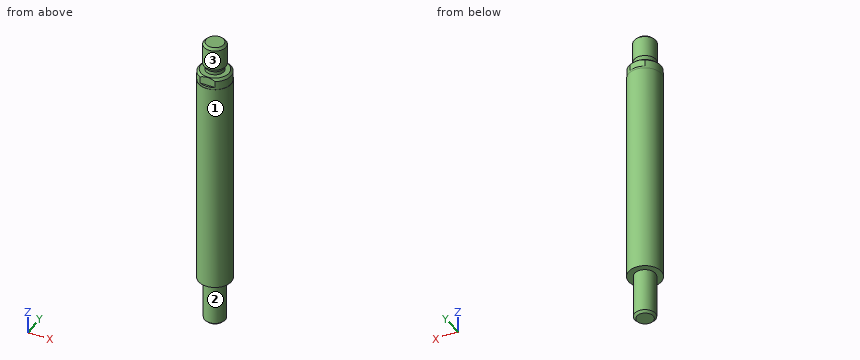
from build123d import *

# Parameters (mm, degrees)
ESQUISSE1_R                   = 15
TIGE_DEPTH                    = 277
ESQUISSE2_OUTSIDE_W           = 88.046
ESQUISSE2_OUTSIDE_H           = 88.046
ESQUISSE2_OUTSIDE_R           = 14.75
CENTRAGE_DE_CHAPE_DEPTH       = 37
ESQUISSE3_OUTSIDE_W           = 88.046
ESQUISSE3_OUTSIDE_H           = 88.046
ESQUISSE3_OUTSIDE_R           = 10
DIAM_TRE_DE_FILETAGE_DEPTH    = 27
ESQUISSE4_OUTSIDE_W           = 88.046
ESQUISSE4_OUTSIDE_H           = 88.046
ESQUISSE4_OUTSIDE_R           = 8.25
GORGE_DE_D_GAGEMENT_DEPTH     = 3
ESQUISSE5_OUTSIDE_W           = 91.51
ESQUISSE5_OUTSIDE_H           = 91.51
ESQUISSE5_OUTSIDE_R           = 8.25
CHANFREIN_DE_D_GAGEMENT_DEPTH = 3
CHANFREIN_DE_D_GAGEMENT_DRAFT = -30
CHANFREIN4_SIZE               = 2
M_PLAT_1_REACH                = 280.815
ESQUISSE6_W                   = 29.5
ESQUISSE6_H                   = 8
ESQUISSE7_OUTSIDE_W           = 88.046
ESQUISSE7_OUTSIDE_H           = 88.046
ESQUISSE7_OUTSIDE_R           = 9.5
CENTRAGE_DE_PISTON_DEPTH      = 42
CHANFREIN_DE_FILETAGE_SIZE    = 2


with BuildPart() as part:
    # Esquisse1 → tige (new body)
    with BuildSketch(Plane.XY):
        with Locations(Location((0, 0, 0), (0, 0, 180))):
            Circle(ESQUISSE1_R)
    extrude(amount=TIGE_DEPTH)

    # Esquisse2 outside → centrage de chape (cut)
    with BuildSketch(Plane.XY.offset(277)):
        Rectangle(ESQUISSE2_OUTSIDE_W, ESQUISSE2_OUTSIDE_H)
        Circle(ESQUISSE2_OUTSIDE_R, mode=Mode.SUBTRACT)
    extrude(amount=-CENTRAGE_DE_CHAPE_DEPTH, mode=Mode.SUBTRACT)

    # Esquisse3 outside → diamètre de filetage (cut)
    with BuildSketch(Plane.XY.offset(277)):
        Rectangle(ESQUISSE3_OUTSIDE_W, ESQUISSE3_OUTSIDE_H)
        Circle(ESQUISSE3_OUTSIDE_R, mode=Mode.SUBTRACT)
    extrude(amount=-DIAM_TRE_DE_FILETAGE_DEPTH, mode=Mode.SUBTRACT)

    # Esquisse4 outside → gorge de d_gagement (cut)
    with BuildSketch(Plane.XY.offset(250)):
        Rectangle(ESQUISSE4_OUTSIDE_W, ESQUISSE4_OUTSIDE_H)
        with Locations(Location((0, 0, 0), (0, 0, 180))):
            Circle(ESQUISSE4_OUTSIDE_R, mode=Mode.SUBTRACT)
    extrude(amount=GORGE_DE_D_GAGEMENT_DEPTH, mode=Mode.SUBTRACT)


with BuildPart() as chanfrein_de_d_gagement_tool:
    # Esquisse5 outside → chanfrein de dégagement (with draft: the straight prism first)
    with BuildSketch(Plane(origin=(0, 0, 253), x_dir=(-1, 0, 0), z_dir=(0, 0, -1))):
        Rectangle(ESQUISSE5_OUTSIDE_W, ESQUISSE5_OUTSIDE_H)
        Circle(ESQUISSE5_OUTSIDE_R, mode=Mode.SUBTRACT)
    extrude(amount=-CHANFREIN_DE_D_GAGEMENT_DEPTH)
    # chanfrein de dégagement: the draft: its side faces are tilted about the plane it starts from
    chanfrein_de_d_gagement_sides = [chanfrein_de_d_gagement_tool.faces().sort_by_distance(p)[0] for p in [
        (0, -45.755, 254.5),
        (-45.755, 0, 254.5),
        (0, 45.755, 254.5),
        (45.755, 0, 254.5),
        (8.25, 0, 254.5),
    ]]
    draft(chanfrein_de_d_gagement_sides, Plane(origin=(0, 0, 253), x_dir=(-1, 0, 0), z_dir=(0, 0, -1)), CHANFREIN_DE_D_GAGEMENT_DRAFT)


with BuildPart() as part_1:
    add(part.part)

    # chanfrein de dégagement: cut by chanfrein_de_d_gagement_tool
    add(chanfrein_de_d_gagement_tool.part, mode=Mode.SUBTRACT)

    # Chanfrein4
    chanfrein4_edges = [part_1.edges().sort_by_distance(p)[0] for p in [
        (-14.75, 0, 250),
        (-10, 0, 277),
    ]]
    chamfer(chanfrein4_edges, length=CHANFREIN4_SIZE)

    # Esquisse6 → méplat 1 (cut, up to next)
    with BuildSketch(Plane(origin=(0, 13, 0), x_dir=(-1, 0, 0), z_dir=(0, 1, 0)), mode=Mode.PRIVATE) as m_plat_1_sk1:
        with Locations((0, 246)):
            Rectangle(ESQUISSE6_W, ESQUISSE6_H)
    m_plat_1_tool1 = extrude(m_plat_1_sk1.sketch, amount=M_PLAT_1_REACH, mode=Mode.PRIVATE) & part_1.part
    m_plat_1 = m_plat_1_tool1.solids().sort_by_distance((0, 13, 246))[0]
    add(m_plat_1, mode=Mode.SUBTRACT)

    # méplat 2: méplat 1 across plane
    add(m_plat_1.mirror(Plane.ZX), mode=Mode.SUBTRACT)

    # Esquisse7 outside → centrage de piston (cut)
    with BuildSketch(Plane(origin=(0, 0, 0), x_dir=(-1, 0, 0), z_dir=(0, 0, -1))):
        Rectangle(ESQUISSE7_OUTSIDE_W, ESQUISSE7_OUTSIDE_H)
        Circle(ESQUISSE7_OUTSIDE_R, mode=Mode.SUBTRACT)
    extrude(amount=-CENTRAGE_DE_PISTON_DEPTH, mode=Mode.SUBTRACT)

    # Chanfrein de filetage
    chanfrein_de_filetage_edges = [part_1.edges().sort_by_distance(p)[0] for p in [
        (9.5, 0, 0),
    ]]
    chamfer(chanfrein_de_filetage_edges, length=CHANFREIN_DE_FILETAGE_SIZE)


solid = part_1.part
Can you work these out from the model? Positions are in its coordinate system, mm. Face numbers are marked on the shaded views. A direction names the side the tool comes from. Round coordinates to 2 decimals unless told otherwise and drop trailing zeros. Loops run counter-clockwise (first coordinate to the right, second up) from the corner with the lowest first, then second, coordinate; pieces in that order, holes last. Notation, with made-up numbers: (3, 14) - (28, 14) arc R18 cw to (28, 23) - close; hole circle Ø1 at (29.5, -20.75). An arc over 180 degrees is marked (long way). Answer in a Markdown table with one row per item. Add a question column.
Q1. Which directions (+Z, -Z, +X, -X, +Y, -Y) give clear straight access to the entire face, cutting with the end or side of a thin tool? Please do the marked faces 1, 2 and 3.
Q2. I need wall thicknesses on L1, parallel to Z at x = 0.75, y = -12.5; L2, parallel to Y at x = 0.25, z = 148.5; L3, parallel to X at y = 1, z = 99. Which ranges of each line are inside material? Lowest first, please.
Q3. For pin 1 Ø6 at (x, z) = (-2.5, 246.5) entering from +Y; pin 2 Ø3 at (x, y) = (8.5, -11.5) entering from +Z; pin 3 Ø8.5 at (x, z) = (1, 248) entering from -Y; pin 4 Ø6 at (x, y) = (-4, -4) entering from -Z, each with a flat end and sliding along its axis, tell me the tip position at first contact or that it passes through.
Q4. I want a section at C-C on z = 129. List the corners of the cut face in (x, y) for me.
A:
| question | item | result |
|---|---|---|
| 1 | face 1 | +Z, -Z |
| 1 | face 2 | -Z |
| 1 | face 3 | +Z |
| 2 | L1 | 42 to 250 |
| 2 | L2 | -15 to 15 |
| 2 | L3 | -14.97 to 14.97 |
| 3 | pin 1 | y = 13 |
| 3 | pin 2 | z = 249.95 |
| 3 | pin 3 | y = -13 |
| 3 | pin 4 | z = 0 |
| 4 | outline | circle Ø30 at (0, 0) |
